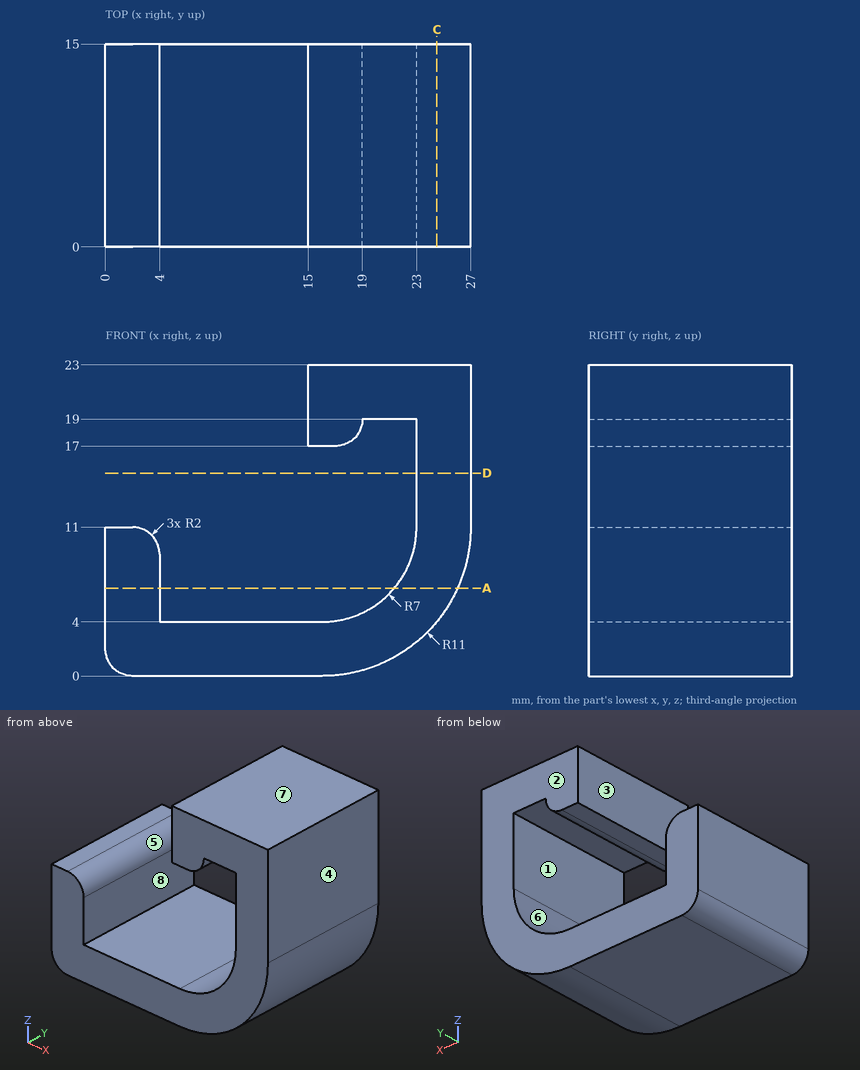
Geometry: see drawing. Coordinates: mm, zero at the bounding-box minimum. A direction names the side the tool comes from. Round coordinates to 2 decimals unless told otherwise and drop trailing zeros. Write each loop counter-clockwise with the first axis right and the second up, starting at its lowest first coordinate (ties: lowest second). Pieces come first, ordered by that corner, then holes.
1) Ray query, L1, parallel to Z at x = 15.75, y = 10.25; L2, parallel to X at y = 4.5, z = 19.75; L3, parallel to X at y = 2, z = 7.5. Return the intervals inside material, ascending.
2) Draft query along Z for the marked faces 6, 7 and 8. Return one class per face: pulls with the +Z half, pulls with the -Z half, needs draft (parallel to the pull), parting line crosses it, or undercut.
3) Contact query for flat-ended pins moving along their axis: P1, Ø1.5, axis at x = 17, z = 6.5, coming from the -Y side; P2, Ø9, axis at y = 4, z = 16, coming from the -X side; P3, Ø5.5, axis at y = 10.5, z = 6, coming from the +X side; P4, Ø1.5, axis at y = 2.5, z = 13, coming from the -X side. Output: stop coordinate, or through.
4) Cut plane A-A (z = 6.5). Return the cut outline in (x, y).
5) Cut plane D-D (z = 15). Return the cut outline in (x, y).
6) Cut plane C-C (x = 24.5). Return the cut outline in (y, z), then the cut area to 3 significant figures.
7) Reachability of the marked faces 1, 2, 3, 4 and 5 from +Z, -Z, +X, -X, +Y, -Y: full face, straight path, thin tool, end or side. Return the list, or none.
Geometry says:
1. L1: z = 0 to 4, 17 to 23
1. L2: x = 15 to 27
1. L3: x = 0 to 4, 22.06 to 26.43
2. face 6: undercut
2. face 7: pulls with the +Z half
2. face 8: needs draft
3. P1: passes through
3. P2: stops at x = 15
3. P3: stops at x = 26.77
3. P4: stops at x = 23
4. outline: (0, 0) - (4, 0) - (4, 15) - (0, 15) - close; (21.36, 0) - (26.04, 0) - (26.04, 15) - (21.36, 15) - close
5. outline: (23, 0) - (27, 0) - (27, 15) - (23, 15) - close
6. outline: (0, 4.02) - (15, 4.02) - (15, 23) - (0, 23) - close
6. area: 285 mm2
7. face 1: +Y, -Y
7. face 2: +Z, -Z, +X, -X, +Y
7. face 3: +Z, -X, +Y, -Y
7. face 4: +Z, -Z, +X, +Y, -Y
7. face 5: +Z, +Y, -Y
